Design review of the part built by this model. Coordinates are the model's own, in mm. Face numbers are marked on the shaded views. A direction names the side the tool comes from. Round coordinates to 2 decimals unless told otherwise and drop trailing zeros. Order: outer loops, then holes, each group sorted by start corner. A loop starts at its lowest first (then second) coordinate and runs counter-clockwise, first axis right, second up. Notation, with made-up numbers: (18, 69.25) - (65, 69.25) arc R15 cw to (65, 82.25) - close; hole circle Ø1 at (5.5, 27). An arc over 180 degrees is marked (long way). Write item = value, one per line.
Autodesk Inventor part; units mm, degrees
ref_plane "YZ Plane" through (0, 0, 0) normal (1, 0, 0) x (0, 1, 0)
ref_plane "XZ Plane" through (0, 0, 0) normal (0, 1, 0) x (-1, 0, 0)
ref_plane "XY Plane" through (0, 0, 0) normal (0, 0, 1) x (1, 0, 0)
sketch "Sketch1" plane through (0, 0, 0) normal (0, 0, 1) x (1, 0, 0)
  line L0 (0, 0) -> (132.5, 0)
  line L1 (132.5, 0) -> (132.5, 10)
  line L2 (132.5, 10) -> (0, 10)
  line L3 (0, 10) -> (0, 0)
  line L4 (132.5, 0) -> (132.5, -20)
  line L5 (132.5, -20) -> (142.5, -20)
  line L6 (142.5, -20) -> (142.5, 10)
  line L7 (142.5, 10) -> (132.5, 10)
  line L8 (0, 0) -> (0, -3)
  line L9 (0, -3) -> (129.5, -3)
  line L10 (129.5, -3) -> (129.5, -20)
  line L11 (129.5, -20) -> (132.5, -20)
  dimension "d0" = 132.5
  dimension "d1" = 10
  dimension "d2" = 10
  dimension "d3" = 20
  dimension "d4" = 3
  dimension "d5" = 3
extrude "Extrusion1" add sketch "Sketch1" along normal blind 3
extrude "Extrusion2" add sketch "Sketch1" against normal blind 10 contours L0 L4 L11 L10 L9 L8
sketch "Sketch2" plane through (0, -3, 3) normal (-1, 0, 0) x (0, 0, 1)
  line L0 (-13, 3) -> (-13, -17)
  line L1 (-13, 3) -> (-3, 12.9668)
  line L2 (-3, 13) -> (-3, 3)
  line L3 (-3, 3) -> (-13, 3)
  line L4 (-13, 0) -> (-13, 3)
  line L5 (-13, 0) -> (0, 0)
  line L6 (0, 13) -> (0, 0)
  line L7 (-3, 13) -> (0, 13)
extrude "Extrusion3" add sketch "Sketch2" along normal blind 3
fillet "Fillet2" radius 2 6 edges at (142.5, 10, 1.5) (142.5, -20, 1.5) (129.5, -20, -3.5) (129.5, -3, -3.5) (-3, 10, 1.5) (-3, -3, -3.5)
properties part number "Z Alignment Guide"
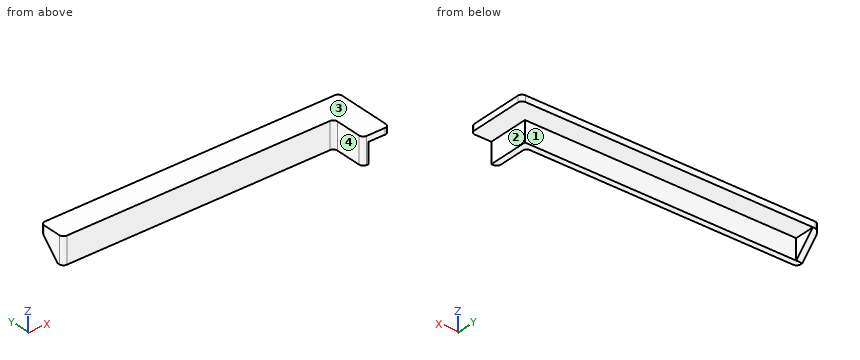
Item 1: For line 1 along Z through (x, y) = (129, 0.75); line 2 along Y through (x, z) = (91, -3); line 3 along Y through (x, z) = (125, 2), list the stretches that pass through material, from the lowest coordinate up. Write a range as [from, to].
Data:
line_1 = [0, 3]
line_2 = [-3, 0]
line_3 = [-3, 10]
Item 2: Take a section at D-D, the plane z = -5.75. State the section outline as (x, y) points.
Data:
outline = (-3, -1) arc R2 ccw to (-1, -3) - (127.5, -3) arc R2 cw to (129.5, -5) - (129.5, -18) arc R2 ccw to (131.5, -20) - (132.5, -20) - (132.5, 0) - (0, 0) - (0, 4.24) - (-3, 4.24) - close
Item 3: For the marked faces 1, 2, 3 and 4, list the 3-axis set-ups (+Z, -Z, +X, -X, +Y, -Y) from which the entire face can be reached by the end or side of a thin tool; tool diameter is ignored.
Data:
face_1 = -Z, +X, +Y
face_2 = -Z, +X, +Y, -Y
face_3 = +Z, +X, -X, +Y, -Y
face_4 = +Z, -Z, -X, -Y
Item 4: Take a section at B-B, the plane y = -7.5. State the section outline as (x, z) points.
Data:
outline = (129.5, -10) - (132.5, -10) - (132.5, 0) - (142.5, 0) - (142.5, 3) - (129.5, 3) - close
Item 5: Take a section at A-A, the plane z = 1.75. State the section outline as (x, y) points.
Data:
outline = (-3, -1) arc R2 ccw to (-1, -3) - (127.5, -3) arc R2 cw to (129.5, -5) - (129.5, -18) arc R2 ccw to (131.5, -20) - (140.5, -20) arc R2 ccw to (142.5, -18) - (142.5, 8) arc R2 ccw to (140.5, 10) - (-1, 10) arc R2 ccw to (-3, 8) - close
Item 6: Insertion check: P1, Ø1.5, axis at x = 108, y = -4.5, coming from the -Z side; P2, Ø2, axis at x = 42, z = 0, coming from the -Y side; P3, Ø1, axis at x = 15, z = -3.5, coming from the +Y side; P4, Ø2, axis at y = -12.5, z = -7.5, coming from the +X side. Each pin has a flat end and moves straight along its axis. Give the tip position at first contact, or say it passes through.
Data:
P1 = through
P2 = -3
P3 = 0
P4 = 132.5
Item 7: Take a section at C-C, the plane x = 48. State the section outline as (y, z) points, and give its area (3 significant figures).
Data:
outline = (-3, -10) - (0, -10) - (0, 0) - (10, 0) - (10, 3) - (-3, 3) - close
area = 69.0 mm2
